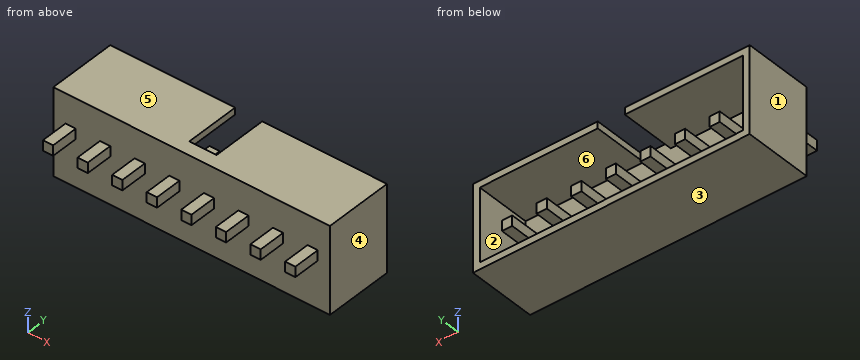
from build123d import *

# Parameters (mm, degrees)
SKETCH_1_W           = 20.32
SKETCH_1_H           = 6.35
EXTRUDE_1_DEPTH      = 5.08
SKETCH_2_W           = 19.32
SKETCH_2_H           = 5.35
CUT_EXTRUDE_1_DEPTH  = 4.08
SKETCH_3_W           = 2
SKETCH_3_H           = 4.08
CUT_EXTRUDE_2_DEPTH  = 1
EXTRUDE_2_DEPTH      = 2
EXTRUDE_2_DEPTH_BACK = 3.58
SKETCH_4_W           = 0.75
SKETCH_4_H           = 0.75


with BuildPart() as part:
    # 草图1 → 拉伸1 (new body)
    with BuildSketch(Plane(origin=(0, 0, 0), x_dir=(1, 0, 0), z_dir=(0, 1, 0))):
        Rectangle(SKETCH_1_W, SKETCH_1_H)
    extrude(amount=EXTRUDE_1_DEPTH)

    # 草图2 → 切除-拉伸1 (cut)
    with BuildSketch(Plane(origin=(0, 5.08, 0), x_dir=(-1, 0, 0), z_dir=(0, 1, 0))):
        Rectangle(SKETCH_2_W, SKETCH_2_H)
    extrude(amount=-CUT_EXTRUDE_1_DEPTH, mode=Mode.SUBTRACT)

    # 草图3 → 切除-拉伸2 (cut)
    with BuildSketch(Plane.XY.offset(3.175)):
        with Locations((0, 3.04)):
            Rectangle(SKETCH_3_W, SKETCH_3_H)
    extrude(amount=-CUT_EXTRUDE_2_DEPTH, mode=Mode.SUBTRACT)

    # 草图4 → 拉伸2 (add, two sides: drawn at the far end of the back side and taken through both)
    with BuildSketch(Plane.XZ.offset(-EXTRUDE_2_DEPTH_BACK)):
        with Locations((-1.27, 0.635)):
            Rectangle(SKETCH_4_W, SKETCH_4_H)
        with Locations((1.27, 0.635)):
            Rectangle(SKETCH_4_W, SKETCH_4_H)
        with Locations((3.81, 0.635)):
            Rectangle(SKETCH_4_W, SKETCH_4_H)
        with Locations((6.35, 0.635)):
            Rectangle(SKETCH_4_W, SKETCH_4_H)
        with Locations((-3.81, 0.635)):
            Rectangle(SKETCH_4_W, SKETCH_4_H)
        with Locations((-6.35, 0.635)):
            Rectangle(SKETCH_4_W, SKETCH_4_H)
        with Locations((-8.89, 0.635)):
            Rectangle(SKETCH_4_W, SKETCH_4_H)
        with Locations((8.89, 0.635)):
            Rectangle(SKETCH_4_W, SKETCH_4_H)
    extrude(amount=EXTRUDE_2_DEPTH + EXTRUDE_2_DEPTH_BACK)


solid = part.part
Part model, mm, in its own coordinate system. Face numbers are marked on the shaded views. A direction names the side the tool comes from. Round coordinates to 2 decimals unless told otherwise and drop trailing zeros. Write each loop counter-clockwise with the first axis right and the second up, starting at its lowest first coordinate (ties: lowest second). Pieces come first, ordered by that corner, then holes. Notation, with made-up numbers: M -8,12 L 24,12 A7 ccw 24,24 Z; hole C -32.5,4 d11. An arc over 180 degrees is marked long. Return JSON: item names as keys, results as strings. Group by question number.
(1) Saw through at C-C on z = -1. Write the cut outline in (x, y).
(2) Saw through at A-A on y = -0.75. Count the separate pieces of the cut face and the enclosed holes in it, then the cut area to 3 significant figures.
(3) Pin check, flat tips, straight feed: pin 1 Ø0.8 at (y, z) = (-0.5, 0.5) entering from +X (3 decimals); pin 2 Ø0.8 at (x, y) = (-3.5, -1.5) entering from +Z. Stop position of each tip, or through.
(4) Which spindle directions (+Z, -Z, +X, -X, +Y, -Y) get a long thin tool onto all of the face, cutting with end or side? Do the marked faces 5 and 6. Say none if no direction does.
(5) Saw through at B-B on x = 0. Write the cut outline in (y, z) (3 decimals), then the cut area to 3 significant figures.
(6) Two-plate mould, pull along X, no slides. Class the marked faces 1, 2, 3 and 4: +X half, -X half, draft (parallel to the pull), parting line (faces both ways), or undercut.
(7) Saw through at D-D on y = 4.75. Write the cut outline in (x, z) (3 decimals), then the cut area to 3 significant figures.
(8) Drill centre lines: probe 1 along Z at (x, y) = (8.75, 3.25) (3 decimals); probe 2 along Z at (x, y) = (4.75, 2.5) (3 decimals); probe 3 along X at (y, z) = (3, 1.25). Where is each one in solid material? Low to high.
Returned:
{
 "1": {"outline": "M -10.16,0 L 10.16,0 L 10.16,5.08 L 9.66,5.08 L 9.66,1 L -9.66,1 L -9.66,5.08 L -10.16,5.08 Z"},
 "2": {"separate pieces": "8", "enclosed holes": "0", "area": "4.50 mm²"},
 "3": {"pin 1": "x = 9.265", "pin 2": "z = 1.01"},
 "4": {"face 5": "+Z, +X, -X, +Y, -Y", "face 6": "+Y"},
 "5": {"outline": "M 0,-3.175 L 5.08,-3.175 L 5.08,-2.675 L 1,-2.675 L 1,3.175 L 0,3.175 Z", "area": "8.39 mm²"},
 "6": {"face 1": "-X half", "face 2": "undercut", "face 3": "draft", "face 4": "+X half"},
 "7": {"outline": "M -10.16,-3.175 L 10.16,-3.175 L 10.16,3.175 L 1,3.175 L 1,2.675 L 9.66,2.675 L 9.66,-2.675 L -9.66,-2.675 L -9.66,2.675 L -1,2.675 L -1,3.175 L -10.16,3.175 Z", "area": "24.7 mm²"},
 "8": {"probe 1": "-3.175 to -2.675, 0.26 to 1.01, 2.675 to 3.175", "probe 2": "-3.175 to -2.675, 2.675 to 3.175", "probe 3": "-10.16 to -9.66, 9.66 to 10.16"}
}
